Geometry: final body of the model. Coordinates: model frame, mm. A direction names the side the tool comes from. Give positions to 0.01 mm unless a question says otherwise; leave off trailing zeros. Write each loop counter-clockwise with the first axis right and the second up, starting at its lowest first coordinate (ties: lowest second). Pieces come first, ordered by that corner, then holes. Notation, with made-up numbers: (7.5, -23.75) -> (39.5, -23.75) arc R22 cw to (39.5, -5.75) -> close; hole circle Ø8 at (-24.75, 43). An arc over 180 degrees is marked (long way). Answer as a JSON object with one key per item and string values.
from build123d import *

# Parameters (mm, degrees)
SKETCH1_R                      = 21.5
BOSS_EXTRUDE1_DEPTH            = 15
TAP_DRILL_FOR_M4X0_7_TAP1_D    = 3.3
BOSS_EXTRUDE2_DEPTH            = 15
SKETCH6_R                      = 11
CUT_EXTRUDE1_DEPTH             = 47.357307946
FILLET1_DEPTH                  = 15
FILLET2_R                      = 10
CBORE_FOR_M4_SHCS2_D           = 4.5
CBORE_FOR_M4_SHCS2_CBORE_D     = 8
CBORE_FOR_M4_SHCS2_CBORE_DEPTH = 4


with BuildPart() as part:
    # Sketch1 → Boss-Extrude1 (new body)
    with BuildSketch(Plane.XY):
        Circle(SKETCH1_R)
    extrude(amount=BOSS_EXTRUDE1_DEPTH)

    # Tap Drill for M4x0.7 Tap1 (through all)
    with Locations(Plane(origin=(0, 0, 0), x_dir=(-1, 0, 0), z_dir=(0, 0, -1))):
        with Locations((0, 16), (16, 0), (0, -16), (-16, 0)):
            Hole(TAP_DRILL_FOR_M4X0_7_TAP1_D / 2)

    # Sketch3 → Boss-Extrude2 (add)
    with BuildSketch(Plane(origin=(0, 0, 0), x_dir=(-1, 0, 0), z_dir=(0, 0, -1))):
        with BuildLine():
            Line((-2.307900214, 25.897366597), (-0.836682642, 21.483713882))
            ThreePointArc((-0.836682642, 21.483713882), (-6.798896971, 20.396690908), (-12.220882218, 17.688980689))
            Line((-12.220882218, 17.688980689), (-13.69209979, 22.102633403))
            ThreePointArc((-13.69209979, 22.102633403), (-9.897366599, 29.692099788), (-2.307900214, 25.897366597))
        make_face()
        with BuildLine():
            Line((17.366563149, 21.316718426), (14.599655804, 15.782903738))
            ThreePointArc((14.599655804, 15.782903738), (9.615092305, 19.230184606), (3.866529512, 21.149466885))
            Line((3.866529512, 21.149466885), (6.633436857, 26.683281574))
            ThreePointArc((6.633436857, 26.683281574), (14.683281576, 29.366563146), (17.366563149, 21.316718426))
        make_face()
        with BuildLine():
            Line((23.846125524, 15.600073637), (17.115813542, 13.011492105))
            ThreePointArc((17.115813542, 13.011492105), (20.066930533, 7.718050205), (21.423562493, 1.811344831))
            Line((21.423562493, 1.811344831), (28.153874476, 4.399926363))
            ThreePointArc((28.153874476, 4.399926363), (31.600073637, 12.153874476), (23.846125524, 15.600073637))
        make_face()
        with BuildLine():
            Line((23.846125524, -15.600073637), (17.115813542, -13.011492105))
            ThreePointArc((17.115813542, -13.011492105), (20.066930533, -7.718050205), (21.423562493, -1.811344831))
            Line((21.423562493, -1.811344831), (28.153874476, -4.399926363))
            ThreePointArc((28.153874476, -4.399926363), (31.600073637, -12.153874476), (23.846125524, -15.600073637))
        make_face()
        with BuildLine():
            Line((17.366563149, -21.316718426), (14.599655804, -15.782903738))
            ThreePointArc((14.599655804, -15.782903738), (9.615092305, -19.230184606), (3.866529512, -21.149466885))
            Line((3.866529512, -21.149466885), (6.633436857, -26.683281574))
            ThreePointArc((6.633436857, -26.683281574), (14.683281576, -29.366563146), (17.366563149, -21.316718426))
        make_face()
        with BuildLine():
            Line((-2.307900214, -25.897366597), (-0.836682642, -21.483713882))
            ThreePointArc((-0.836682642, -21.483713882), (-6.798896971, -20.396690908), (-12.220882218, -17.688980689))
            Line((-12.220882218, -17.688980689), (-13.69209979, -22.102633403))
            ThreePointArc((-13.69209979, -22.102633403), (-9.897366599, -29.692099788), (-2.307900214, -25.897366597))
        make_face()
    extrude(amount=-BOSS_EXTRUDE2_DEPTH)

    # Sketch6 → Cut-Extrude1 (cut, through all)
    with BuildSketch(Plane(origin=(0, 0, 0), x_dir=(-1, 0, 0), z_dir=(0, 0, -1))):
        Circle(SKETCH6_R)
    extrude(amount=-CUT_EXTRUDE1_DEPTH, mode=Mode.SUBTRACT)

    # Fillet1: read off the stored shape, not the designer's step
    # Fillet1 outline → Fillet1 (add)
    with BuildSketch(Plane.XY):
        with BuildLine():
            ThreePointArc((13.744239295, -25.733122887), (16.656803279, -16.794634864), (19.959130827, -7.9926902))
            ThreePointArc((19.959130827, -7.9926902), (16.804547664, -13.411084139), (12.220882218, -17.688980689))
            Line((12.220882218, -17.688980689), (13.69209979, -22.102633403))
            ThreePointArc((13.69209979, -22.102633403), (13.999381334, -23.913839504), (13.744239295, -25.733122887))
        make_face()
        with BuildLine():
            ThreePointArc((12.220882218, 17.688980689), (16.804547664, 13.411084139), (19.959130827, 7.9926902))
            ThreePointArc((19.959130827, 7.9926902), (16.656803279, 16.794634864), (13.744239295, 25.733122887))
            ThreePointArc((13.744239295, 25.733122887), (13.999381334, 23.913839504), (13.69209979, 22.102633403))
            Line((13.69209979, 22.102633403), (12.220882218, 17.688980689))
        make_face()
        with BuildLine():
            ThreePointArc((-1.269568391, -24.771937297), (1.604087257, -26.779090443), (4.4444823, -28.833041886))
            ThreePointArc((4.4444823, -28.833041886), (3.148798639, -27.530700404), (2.307900214, -25.897366597))
            Line((2.307900214, -25.897366597), (0.836682642, -21.483713882))
            ThreePointArc((0.836682642, -21.483713882), (-1.524113932, -21.445910489), (-3.866529512, -21.149466885))
            Line((-3.866529512, -21.149466885), (-6.633436857, -26.683281574))
            ThreePointArc((-6.633436857, -26.683281574), (-7.59800708, -28.077064913), (-8.913884182, -29.145472684))
            ThreePointArc((-8.913884182, -29.145472684), (-5.114227359, -26.919376327), (-1.269568391, -24.771937297))
        make_face()
        with BuildLine():
            ThreePointArc((2.307900214, 25.897366597), (3.148798639, 27.530700404), (4.4444823, 28.833041886))
            ThreePointArc((4.4444823, 28.833041886), (1.604087257, 26.779090443), (-1.269568391, 24.771937297))
            ThreePointArc((-1.269568391, 24.771937297), (-5.114227359, 26.919376327), (-8.913884182, 29.145472684))
            ThreePointArc((-8.913884182, 29.145472684), (-7.59800708, 28.077064913), (-6.633436857, 26.683281574))
            Line((-6.633436857, 26.683281574), (-3.866529512, 21.149466885))
            ThreePointArc((-3.866529512, 21.149466885), (-1.524113932, 21.445910489), (0.836682642, 21.483713882))
            Line((0.836682642, 21.483713882), (2.307900214, 25.897366597))
        make_face()
        with BuildLine():
            ThreePointArc((-18.827219, -17.493972554), (-18.367768434, -21.052580188), (-17.968047643, -24.618390952))
            ThreePointArc((-17.968047643, -24.618390952), (-17.902847687, -22.924644608), (-17.366563149, -21.316718426))
            Line((-17.366563149, -21.316718426), (-14.599655804, -15.782903738))
            ThreePointArc((-14.599655804, -15.782903738), (-15.918163511, -14.452061114), (-17.115813542, -13.011492105))
            Line((-17.115813542, -13.011492105), (-23.846125524, -15.600073637))
            ThreePointArc((-23.846125524, -15.600073637), (-25.412904992, -15.971207537), (-27.021964079, -15.912325213))
            ThreePointArc((-27.021964079, -15.912325213), (-22.91688029, -16.663195777), (-18.827219, -17.493972554))
        make_face()
        with BuildLine():
            ThreePointArc((-17.366563149, 21.316718426), (-17.902847687, 22.924644608), (-17.968047643, 24.618390952))
            ThreePointArc((-17.968047643, 24.618390952), (-18.367768434, 21.052580188), (-18.827219, 17.493972554))
            ThreePointArc((-18.827219, 17.493972554), (-22.91688029, 16.663195777), (-27.021964079, 15.912325213))
            ThreePointArc((-27.021964079, 15.912325213), (-25.412904992, 15.971207537), (-23.846125524, 15.600073637))
            Line((-23.846125524, 15.600073637), (-17.115813542, 13.011492105))
            ThreePointArc((-17.115813542, 13.011492105), (-15.918163511, 14.452061114), (-14.599655804, 15.782903738))
            Line((-14.599655804, 15.782903738), (-17.366563149, 21.316718426))
        make_face()
        with BuildLine():
            ThreePointArc((-25.965184624, 0), (-28.313790974, -3.170063395), (-30.720438686, -6.296291235))
            ThreePointArc((-30.720438686, -6.296291235), (-29.565542777, -5.174349297), (-28.153874476, -4.399926363))
            Line((-28.153874476, -4.399926363), (-21.423562493, -1.811344831))
            ThreePointArc((-21.423562493, -1.811344831), (-21.5, 0), (-21.423562493, 1.811344831))
            Line((-21.423562493, 1.811344831), (-28.153874476, 4.399926363))
            ThreePointArc((-28.153874476, 4.399926363), (-29.565542777, 5.174349297), (-30.720438686, 6.296291235))
            ThreePointArc((-30.720438686, 6.296291235), (-28.313790974, 3.170063395), (-25.965184624, 0))
        make_face()
    extrude(amount=FILLET1_DEPTH)

    # Fillet2
    fillet2_edges = [part.edges().sort_by_distance(p)[0] for p in [
        (-1.269568391, -24.771937297, 7.5),
        (-18.827219, -17.493972554, 7.5),
        (-25.965184624, 0, 7.5),
        (-18.827219, 17.493972554, 7.5),
        (-1.269568391, 24.771937297, 7.5),
    ]]
    fillet(fillet2_edges, radius=FILLET2_R)

    # CBORE for M4 SHCS2 (through all)
    with Locations(Plane.XY.offset(15)):
        with Locations((8.000000002, 24), (-12.000000003, 24), (-26, 10), (-26, -10), (-12.000000003, -24), (8.000000002, -24)):
            CounterBoreHole(CBORE_FOR_M4_SHCS2_D / 2, CBORE_FOR_M4_SHCS2_CBORE_D / 2, CBORE_FOR_M4_SHCS2_CBORE_DEPTH)


solid = part.part
Q1. First-contact query: P1, Ø6, axis at x = -14, z = 5.5, coming from the +Y side; P2, Ø3, axis at x = 3, z = 12, coming from the +Y side; P3, Ø3, axis at x = 1.5, z = 6, coming from the -Y side; P4, Ø4, axis at x = -27, y = 9.5, coming from the +Z side. Flat tips, straight axial feed; report the tip coordinate or a pass-through.
Values:
{"P1": "y = 30", "P2": "y = 28.87", "P3": "y = -27.87", "P4": "z = 11"}
Q2. Cut plane B-B (y = 0). State how many separate pieces and enclosed holes the cut face has, and give its area (3 significant figures).
Values:
{"separate pieces": "4", "enclosed holes": "0", "area": "321 mm²"}
Q3. Mould query, pull axis Y, two halves, no side actions, for faces 1 (the flat face through (-12, 0, 0)), 2 (the cylindrical face through (-14.563, 29.425, 7.395)), 3 (the cylindrical face through (-11.512, 21.804, 5.423)). Classes: pulls with the +Y half, pulls with the -Y half, needs draft (parallel to the pull), parting line crosses it, or undercut.
Values:
{"face 1": "needs draft", "face 2": "pulls with the +Y half", "face 3": "undercut"}
Q4. Cut plane A-A (x = -12). Return the cut outline in (y, z).
Values:
{"outline": "(-30, 0) -> (-26.25, 0) -> (-26.25, 11) -> (-28, 11) -> (-28, 15) -> (-30, 15) -> close; (-21.75, 0) -> (21.75, 0) -> (21.75, 11) -> (20, 11) -> (20, 15) -> (-20, 15) -> (-20, 11) -> (-21.75, 11) -> close; (26.25, 0) -> (30, 0) -> (30, 15) -> (28, 15) -> (28, 11) -> (26.25, 11) -> close"}
Q5. Cut plane D-D (y = -10). Return the cut outline in (x, z), and give its area (3 significant figures).
Values:
{"outline": "(-32, 0) -> (-28.25, 0) -> (-28.25, 11) -> (-30, 11) -> (-30, 15) -> (-32, 15) -> close; (-23.75, 0) -> (-4.58, 0) -> (-4.58, 15) -> (-22, 15) -> (-22, 11) -> (-23.75, 11) -> close; (4.58, 0) -> (19.17, 0) -> (19.17, 15) -> (4.58, 15) -> close", "area": "549 mm²"}
Q6. Set-up query: faces 4 (the flat face through (-24, -12, 11)), 5 (the cylindrical face through (16.7, 16.67, 7.4)). Return all of +Z, -Z, +X, -X, +Y, -Y with unobstructed straight access to the full face (end or side cutting, diameter ignored); none if empty.
Values:
{"face 4": "+Z", "face 5": "+Z, -Z, +X, +Y"}
Q7. Material intervals for L1, parallel to Y at x = -12, z = 5; L2, parallel to X at y = -26.5, z = 14; L3, parallel to Y at x = -26, z = 7.5, sorted ascending. Write a range as from..to.
Values:
{"L1": "-30..-26.25, -21.75..21.75, 26.25..30", "L2": "-17.45..-15.12, -8.88..4.88, 11.12..13.45", "L3": "-16.09..-12.25, -7.75..7.75, 12.25..16.09"}
